Work out the finished part from the listing and answer in its coordinate system (mm). Face numbers are marked on the shaded views. Coordinates: 2 decimals unless noted, no trailing zeros. Order: outer loops, then holes, each group sorted by start corner. A loop starts at its lowest first (then second) coordinate and runs counter-clockwise, first axis right, second up.
1. The part is cut by section D-D, the plane x = -8. Give the vertices of the cut face in (y, z).
2. Determine the mould class of the marked faces 1, 2 and 3 for opening direction Z: +Z half, -Z half, draft (parallel to the pull), parting line (faces both ways), or undercut.
3. The part is cut by section C-C, the plane x = 0. Give the vertices of the cut face in (y, z), then the cut area to 3 significant figures.
4. The part is cut by section B-B, the plane z = 0. Give the vertices of the cut face in (x, y).
5. The part is cut by section A-A, the plane y = 3.75. Give the vertices of the cut face in (x, z), then the cut area to 3 significant figures.
6. Flat-ended cylindrical pins translate along their axes: pin 1 Ø8 at (x, z) = (0, 0) entering from -Y; pin 2 Ø1 at (x, y) = (3.5, 3) entering from -Z; pin 3 Ø1.5 at (x, y) = (2.5, 1.5) entering from -Z; pin 4 Ø1 at (y, z) = (4, 18.5) entering from -X. Find the tip coordinate at first contact, or state that the pin passes through.
7. Find the intervals of material crossed by probe 1 along Z at (x, y) = (0, 4.25); probe 2 along Z at (x, y) = (-1.75, 7.75); probe 3 along X at (y, z) = (6.25, 16), in increasing order.
Autodesk Inventor part; units mm, degrees
ref_plane "YZ Plane" through (0, 0, 0) normal (1, 0, 0) x (0, 1, 0)
ref_plane "XZ Plane" through (0, 0, 0) normal (0, 1, 0) x (-1, 0, 0)
ref_plane "XY Plane" through (0, 0, 0) normal (0, 0, 1) x (1, 0, 0)
sketch "Block1" plane through (0, 0, 0) normal (0, 0, 1) x (1, 0, 0)
  circle A0 centre (0, 0) radius 20.22
  circle A1 centre (0, 12) radius 2.72
  circle A2 centre (0, 0) radius 5.22
  circle A3 centre (0, -12) radius 2.72
sketch "Block2" plane through (0, 0, 0) normal (0, 0, 1) x (1, 0, 0)
  circle A0 centre (0, 0) radius 22.72
  circle A1 centre (-12, 12) radius 2.72
  circle A2 centre (0, 0) radius 5.22
  point P0 (-4, 4)
sketch "Block3" plane through (0, 0, 0) normal (0, 0, 1) x (1, 0, 0)
  line L0 (-10.22, -16.9706) -> (-10.22, 16.9706)
  arc A0 (10.22, 16.9706) -> (-10.22, 16.9706) centre (0, 16.9706) ccw
  line L1 (10.22, 16.9706) -> (10.22, -16.9706)
  arc A1 (-10.22, -16.9706) -> (10.22, -16.9706) centre (0, -16.9706) ccw
  circle A2 centre (0, -16.9706) radius 2.72
  circle A3 centre (0, 0) radius 5.22
  circle A4 centre (0, 16.9706) radius 2.72
  point P0 (0, 0)
sketch "Sketch9" plane through (0, 0, 0) normal (0, 1, 0) x (-1, 0, 0)
  line L0 (0, -16.9706) -> (0, 16.9706) construction
  line L1 (10, -16.9706) -> (10, 16.9706)
  line L2 (-10, 16.9706) -> (-10, -16.9706)
  arc A0 (-10, -16.9706) -> (10, -16.9706) centre (0, -16.9706) ccw
  arc A1 (10, 16.9706) -> (-10, 16.9706) centre (0, 16.9706) ccw
  circle A2 centre (0, 0) radius 5
  circle A3 centre (0, 16.9706) radius 2.5
  circle A4 centre (0, -16.9706) radius 2.5
  dimension "d33" = 10
  dimension "d34" = 33.9411
  dimension "d35" = 10
  dimension "d36" = 5
  dimension "d37" = 5
extrude "Extrusion6" add sketch "Sketch9" along normal blind 10
sketch "Sketch10" plane through (0, 10, 0) normal (0, 1, 0) x (1, 0, 0)
  circle A0 centre (0, 0) radius 5
  circle A1 centre (0, 16.9706) radius 2.5
  circle A2 centre (0, -16.9706) radius 2.5
  line L0 (-10, 16.9706) -> (-10, -16.9706)
  arc A3 (-10, -16.9706) -> (10, -16.9706) centre (0, -16.9706) ccw
  line L1 (10, -16.9706) -> (10, 16.9706)
  arc A4 (10, 16.9706) -> (-10, 16.9706) centre (0, 16.9706) ccw
sketch "DXF" plane through (0, 0, 0) normal (0, 1, 0) x (-1, 0, 0)
  point P0 (0, 0)
properties part number "gearSupport"
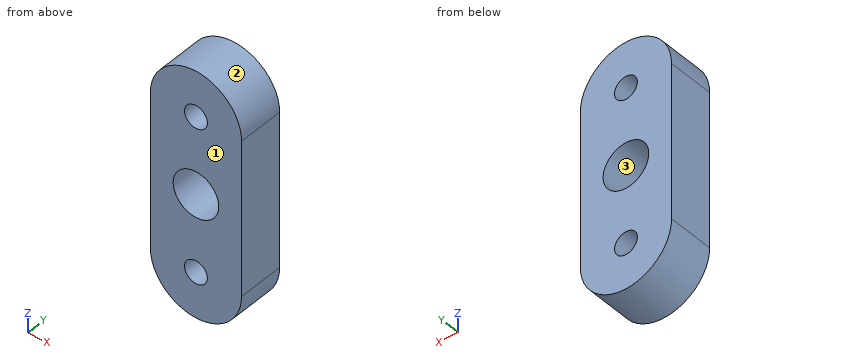
Geometry says:
1. outline: (0, -22.97) - (10, -22.97) - (10, 22.97) - (0, 22.97) - close
2. face 1: draft
2. face 2: +Z half
2. face 3: undercut
3. outline: (0, -26.97) - (10, -26.97) - (10, -19.47) - (0, -19.47) - close; (0, -14.47) - (10, -14.47) - (10, -5) - (0, -5) - close; (0, 5) - (10, 5) - (10, 14.47) - (0, 14.47) - close; (0, 19.47) - (10, 19.47) - (10, 26.97) - (0, 26.97) - close
3. area: 339 mm2
4. outline: (-10, 0) - (-5, 0) - (-5, 10) - (-10, 10) - close; (5, 0) - (10, 0) - (10, 10) - (5, 10) - close
5. outline: (-10, -16.97) arc R10 ccw to (10, -16.97) - (10, 16.97) arc R10 ccw to (-10, 16.97) - close; hole circle Ø10 at (0, 0); hole circle Ø5 at (0, -16.97); hole circle Ø5 at (0, 16.97)
5. area: 875 mm2
6. pin 1: passes through
6. pin 2: stops at z = -26.51
6. pin 3: stops at z = -26.82
6. pin 4: stops at x = -9.95
7. probe 1: z = -26.97 to -19.47, -14.47 to -5, 5 to 14.47, 19.47 to 26.97
7. probe 2: z = -26.82 to -18.76, -15.19 to -4.68, 4.68 to 15.19, 18.76 to 26.82
7. probe 3: x = -10 to -2.3, 2.3 to 10
